from build123d import *

# Parameters (mm, degrees)
SKETCH1_W           = 9.525
SKETCH1_H           = 6.35
BOSS_EXTRUDE1_DEPTH = 1.5875
SKETCH2_R           = 1.5875
SKETCH2_W           = 1.5875
SKETCH2_H           = 6.35
BOSS_EXTRUDE2_DEPTH = 6.35


with BuildPart() as part:
    # Sketch1 → Boss-Extrude1 (new body)
    with BuildSketch(Plane(origin=(0, 0, 0), x_dir=(1, 0, 0), z_dir=(0, 1, 0))):
        Rectangle(SKETCH1_W, SKETCH1_H)
    extrude(amount=BOSS_EXTRUDE1_DEPTH)

    # Sketch2 → Boss-Extrude2 (add)
    with BuildSketch(Plane(origin=(0, 1.5875, 0), x_dir=(1, 0, 0), z_dir=(0, 1, 0))):
        with Locations((-2.38125, 0)):
            Circle(SKETCH2_R)
        with Locations((3.96875, 0)):
            Rectangle(SKETCH2_W, SKETCH2_H)
    extrude(amount=BOSS_EXTRUDE2_DEPTH)


solid = part.part
Input: part model. Units: mm. Frame: model coordinates. A direction names the side the tool comes from. Give positions to 0.01 mm unless a question says otherwise; leave off trailing zeros. Loops run counter-clockwise (first coordinate to the right, second up) from the corner with the lowest first, then second, coordinate; pieces in that order, holes last. Notation, with made-up numbers: M 78.5,-13.5 L 90.5,-13.5 A14 ccw 90.5,-8.5 Z; hole C -11.5,49 d2. An arc over 180 degrees is marked long. Use CSV: the item, a comma, the result in double quotes.
(1) Material intervals for L1, parallel to Y at x = -1.25, z = 3; L2, parallel to X at y = 7.5, z = 0.75 (1 decimal); L3, parallel to X at y = 2.75, z = -1 (1 decimal), sorted ascending. Write a range as [from, to].
Outcome:
L1,"y = [0, 1.59]"
L2,"x = [-3.8, -1], [3.2, 4.8]"
L3,"x = [-3.6, -1.1], [3.2, 4.8]"
(2) Section C-C, the plane x = 3. Return loops of the section in (y, z) (1 decimal), plus the area to 3 significant figures.
Outcome:
outline,"M 0,-3.2 L 1.6,-3.2 L 1.6,3.2 L 0,3.2 Z"
area,"10.1 mm²"
(3) Section D-D, the plane z = 0. Return loops of the section in (x, y) (1 decimal), plus the area to 3 significant figures.
Outcome:
outline,"M -4.8,0 L 4.8,0 L 4.8,7.9 L 3.2,7.9 L 3.2,1.6 L -0.8,1.6 L -0.8,7.9 L -4,7.9 L -4,1.6 L -4.8,1.6 Z"
area,"45.4 mm²"
(4) Set-up query: faces 5 (the face through (-0.87, 4.72, -0.48)), 6 (the face through (1, 1, 3.175)), 7 (the face through (3.175, 5, 0)). Return all of +Z, -Z, +X, -X, +Y, -Y with unobstructed straight access to the full face (end or side cutting, diameter ignored); none if empty.
Outcome:
face 5,"+Y"
face 6,"+Z, +X, -X, +Y, -Y"
face 7,"+Z, -Z, +Y"
(5) Pull-direction query (X, two-part tool) for faces 1 (the face through (4.762, 4, 0)), 2 (the face through (-2, 7.938, 0)), 3 (the face through (-4.762, 1, 0)), 4 (the face through (0, 1.588, 0)); classes: pulls with the +X half, pulls with the -X half, needs draft (parallel to the pull), parting line crosses it, or undercut.
Outcome:
face 1,"pulls with the +X half"
face 2,"needs draft"
face 3,"pulls with the -X half"
face 4,"undercut"
(6) Section A-A, the plane y = 5. Return loops of the section in (x, z) (1 decimal).
Outcome:
outline,"C -2.4,0 d3.2; M 3.2,-3.2 L 4.8,-3.2 L 4.8,3.2 L 3.2,3.2 Z"
(7) Section B-B, the plane z = 1.75. Return loops of the section in (x, y) (1 decimal), plus the area to 3 significant figures.
Outcome:
outline,"M -4.8,0 L 4.8,0 L 4.8,7.9 L 3.2,7.9 L 3.2,1.6 L -4.8,1.6 Z"
area,"25.2 mm²"
(8) Pin query (flat end, axial travel): P1, Ø3, axis at x = -2.5, y = 5, coming from the +Z side; P2, Ø1.5, axis at y = 5, z = 2, coming from the -X side. Return the tip coordinate at first contact, or that it passes through.
Outcome:
P1,"stops at z = 1.59"
P2,"stops at x = -3.36"
